```python
from build123d import *

# Parameters (mm, degrees)
BOSS_EXTRUDE1_DEPTH = 5.5
SKETCH2_R           = 1.65
CUT_EXTRUDE1_DEPTH  = 5.5
BOSS_EXTRUDE2_DEPTH = 3
CUT_EXTRUDE2_DEPTH  = 2.75
SKETCH5_R           = 1.95
SKETCH5_R_2         = 1.35
SKETCH5_R_3         = 1.15
SKETCH5_R_4         = 2
CUT_EXTRUDE3_DEPTH  = 4.3
SKETCH7_R           = 1.95
SKETCH7_R_2         = 1.35
CUT_EXTRUDE4_DEPTH  = 3
CHAMFER1_SIZE       = 1
CUT_EXTRUDE5_DEPTH  = 2.75


with BuildPart() as part:
    # Sketch1 → Boss-Extrude1 (new body)
    with BuildSketch(Plane(origin=(0, 0, 0), x_dir=(1, 0, 0), z_dir=(0, 1, 0))):
        with BuildLine():
            Line((-7.755996733, 16.049992949), (-18.008818061, 22.554712546))
            ThreePointArc((-18.008818061, 22.554712546), (-25.669699487, 29.278547542), (-27.75, 19.3))
            Line((-27.75, 19.3), (-27.75, 8.1))
            Line((-27.75, 8.1), (-21.75, 2.8))
            Line((-21.75, 2.8), (-21.75, 0))
            Line((-21.75, 0), (21.75, 0))
            Line((21.75, 0), (21.75, 7))
            Line((21.75, 7), (18.25, 11))
            Line((18.25, 11), (-5.907756778, 15.263133549))
            ThreePointArc((-5.907756778, 15.263133549), (-6.75113203, 15.846223088), (-7.755996733, 16.049992949))
        make_face()
        with BuildLine():
            Line((-19.85, 18.630440726), (-10.05956754, 12.419075498))
            ThreePointArc((-10.05956754, 12.419075498), (-8.75757921, 11.15750472), (-6.94630287, 11.079964685))
            Line((-6.94630287, 11.079964685), (-0.119008465, 9.875148026))
            Line((-0.119008465, 9.875148026), (2.380991535, 6.875148026))
            Line((2.380991535, 6.875148026), (2.380991535, 1.3))
            Line((2.380991535, 1.3), (-12.151886792, 1.3))
            Line((-12.151886792, 1.3), (-19.85, 8.1))
            Line((-19.85, 8.1), (-19.85, 18.630440726))
        make_face(mode=Mode.SUBTRACT)
    extrude(amount=BOSS_EXTRUDE1_DEPTH)

    # Sketch2 → Cut-Extrude1 (cut)
    with BuildSketch(Plane(origin=(0, 5.5, 0), x_dir=(1, 0, 0), z_dir=(0, 1, 0))):
        with Locations(Location((-7.75, 13.5, 0), (0, 0, 270))):
            Circle(SKETCH2_R)
    extrude(amount=-CUT_EXTRUDE1_DEPTH, mode=Mode.SUBTRACT)

    # Sketch3 → Boss-Extrude2 (add)
    with BuildSketch(Plane(origin=(0, 5.5, 0), x_dir=(1, 0, 0), z_dir=(0, 1, 0))):
        with BuildLine():
            ThreePointArc((-27.75, 19.3), (-23.8, 17.782636193), (-19.85, 19.3))
            ThreePointArc((-19.85, 19.3), (-18.664735174, 20.777631), (-18.008818061, 22.554712546))
            ThreePointArc((-18.008818061, 22.554712546), (-17.927267525, 23.116055854), (-17.9, 23.682636193))
            ThreePointArc((-17.9, 23.682636193), (-26.198436991, 29.073137097), (-27.75, 19.3))
        make_face()
        with BuildLine():
            Line((-12.151886792, 1.3), (-19.85, 8.1))
            Line((-19.85, 8.1), (-19.85, 18.630440726))
            Line((-19.85, 18.630440726), (-19.85, 19.3))
            ThreePointArc((-19.85, 19.3), (-23.8, 17.782636193), (-27.75, 19.3))
            Line((-27.75, 19.3), (-27.75, 8.1))
            Line((-27.75, 8.1), (-21.75, 2.8))
            Line((-21.75, 2.8), (-21.75, 0))
            Line((-21.75, 0), (21.75, 0))
            Line((21.75, 0), (21.75, 1.3))
            Line((21.75, 1.3), (2.380991535, 1.3))
            Line((2.380991535, 1.3), (-12.151886792, 1.3))
        make_face()
    extrude(amount=BOSS_EXTRUDE2_DEPTH)

    # Sketch4 → Cut-Extrude2 (cut)
    with BuildSketch(Plane.XZ):
        with BuildLine():
            ThreePointArc((-27.75, -19.3), (-29.307610804, -25.798344876), (-23.8, -29.582636193))
            Line((-23.8, -29.582636193), (-23.8, -7.3))
            Line((-23.8, -7.3), (-26.844339623, -7.3))
            Line((-26.844339623, -7.3), (-27.75, -8.1))
            Line((-27.75, -8.1), (-27.75, -19.3))
        make_face()
    extrude(amount=-CUT_EXTRUDE2_DEPTH, mode=Mode.SUBTRACT)

    # Sketch5 → Cut-Extrude3 (cut)
    with BuildSketch(Plane.XZ):
        with Locations(Location((-23.8, -23.682636193, 0), (0, 0, 90))):
            Circle(SKETCH5_R)
        with Locations(Location((-23.8, -13.882636193, 0), (0, 0, 90))):
            Circle(SKETCH5_R_2)
        with Locations(Location((-20, -4.382636193, 0), (0, 0, 270))):
            Circle(SKETCH5_R_3)
        with Locations(Location((15.000589162, -5.5, 0), (0, 0, 270))):
            Circle(SKETCH5_R_4)
    extrude(amount=-CUT_EXTRUDE3_DEPTH, mode=Mode.SUBTRACT)

    # Sketch7 → Cut-Extrude4 (cut)
    with BuildSketch(Plane.XZ.offset(-4.3)):
        with Locations(Location((-23.8, -23.682636193, 0), (0, 0, 90))):
            Circle(SKETCH7_R)
        with Locations(Location((-23.8, -13.882636193, 0), (0, 0, 90))):
            Circle(SKETCH7_R_2)
    extrude(amount=-CUT_EXTRUDE4_DEPTH, mode=Mode.SUBTRACT)

    # Chamfer1
    chamfer1_edges = [part.edges().sort_by_distance(p)[0] for p in [
        (-23.8, 8.5, -29.582636193),
        (-27.75, 8.5, -13.7),
        (-24.75, 8.5, -5.45),
        (-21.75, 8.5, -1.4),
        (-19.85, 8.5, -13.7),
    ]]
    chamfer(chamfer1_edges, length=CHAMFER1_SIZE)

    # Sketch8 → Cut-Extrude5 (cut)
    with BuildSketch(Plane.XZ):
        with BuildLine():
            Line((-21.05, -7.3), (-23.8, -7.3))
            Line((-23.8, -7.3), (-23.8, -12.532636193))
            ThreePointArc((-23.8, -12.532636193), (-22.45, -13.882636193), (-23.8, -15.232636193))
            Line((-23.8, -15.232636193), (-23.8, -18.982636193))
            ThreePointArc((-23.8, -18.982636193), (-22.355013861, -19.210274953), (-21.05, -19.871140424))
            Line((-21.05, -19.871140424), (-21.05, -7.3))
        make_face()
        with BuildLine():
            ThreePointArc((-19.1, -23.682636193), (-19.615803542, -21.54195873), (-21.05, -19.871140424))
            ThreePointArc((-21.05, -19.871140424), (-22.355013861, -19.210274953), (-23.8, -18.982636193))
            Line((-23.8, -18.982636193), (-23.8, -21.732636193))
            ThreePointArc((-23.8, -21.732636193), (-21.85, -23.682636193), (-23.8, -25.632636193))
            Line((-23.8, -25.632636193), (-23.8, -28.382636193))
            ThreePointArc((-23.8, -28.382636193), (-20.476598128, -27.006038065), (-19.1, -23.682636193))
        make_face()
        with BuildLine():
            Line((-23.8, -21.732636193), (-23.8, -18.982636193))
            ThreePointArc((-23.8, -18.982636193), (-28.5, -23.682636193), (-23.8, -28.382636193))
            Line((-23.8, -28.382636193), (-23.8, -25.632636193))
            ThreePointArc((-23.8, -25.632636193), (-21.85, -23.682636193), (-23.8, -21.732636193))
        make_face()
    extrude(amount=-CUT_EXTRUDE5_DEPTH, mode=Mode.SUBTRACT)


solid = part.part
```
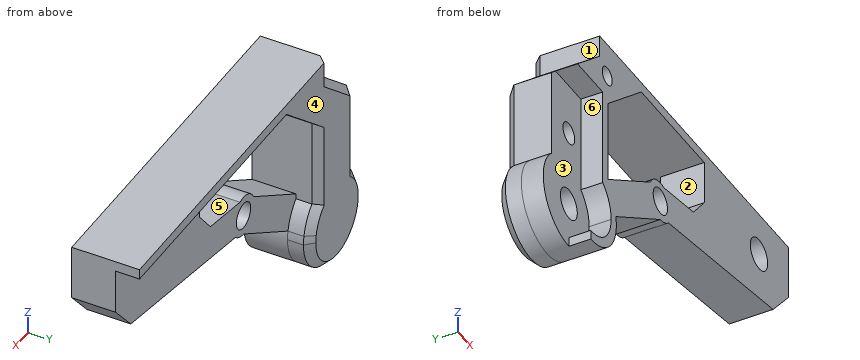
The listing builds one solid part. Answer for the finished solid, in the listing's coordinates (mm). Face numbers are marked on the shaded views. A direction names the side the tool comes from. Give positions to 0.01 mm unless a question says otherwise; leave off trailing zeros. Order: outer loops, then holes, each group sorted by start corner. A loop starts at its lowest first (then second) coordinate and runs counter-clockwise, first axis right, second up.
Item 1: The part is cut by section B-B, the plane y = 1.75. Give the vertices of the cut face in (x, z), and give its area (3 significant figures).
From the geometry:
outline: (-26.84, -7.3) - (-21.05, -7.3) - (-21.05, -19.87) arc R4.7 cw to (-23.8, -28.38) - (-23.8, -29.58) arc R5.9 ccw to (-18.01, -22.55) - (-7.76, -16.05) arc R2.55 ccw to (-5.91, -15.26) - (18.25, -11) - (21.75, -7) - (21.75, 0) - (-21.75, 0) - (-21.75, -2.8) - close; hole circle Ø2.3 at (-20, -4.38); hole (-19.85, -18.63) - (-10.06, -12.42) arc R2.55 cw to (-6.95, -11.08) - (-0.12, -9.88) - (2.38, -6.88) - (2.38, -1.3) - (-12.15, -1.3) - (-19.85, -8.1) - close; hole circle Ø3.3 at (-7.75, -13.5); hole circle Ø4 at (15, -5.5)
area: 420 mm2
Item 2: The part is cut by section A-A, the plane z = -13.5. Give the vertices of the cut face in (x, y), and give its area (3 significant figures).
From the geometry:
outline: (-27.75, 2.75) - (-25.09, 2.75) - (-25.09, 7.3) - (-22.51, 7.3) - (-22.51, 2.75) - (-21.05, 2.75) - (-21.05, 0) - (-19.85, 0) - (-19.85, 7.5) - (-20.85, 8.5) - (-26.75, 8.5) - (-27.75, 7.5) - close; (-11.76, 0) - (-9.4, 0) - (-9.4, 5.5) - (-11.76, 5.5) - close; (-6.1, 0) - (4.08, 0) - (4.08, 5.5) - (-6.1, 5.5) - close
area: 105 mm2
Item 3: The part is cut by section C-C, the plane x = 5.5. Give the vertices of the cut face in (y, z).
From the geometry:
outline: (0, -13.25) - (5.5, -13.25) - (5.5, -1.3) - (8.5, -1.3) - (8.5, 0) - (0, 0) - close
Item 4: Find the intervals of material crossed by probe 1 along Z at (x, y) = (-23.8, 4.35); probe 2 along X at (y, z) = (6.5, -23.5); probe 3 along Y at (x, z) = (-10.5, -12.75), in increasing order.
From the geometry:
probe 1: z = -29.58 to -25.63, -21.73 to -15.23, -12.53 to -4.61
probe 2: x = -29.7 to -25.74, -21.86 to -17.9
probe 3: y = 0 to 5.5
Item 5: Given pin 1 Ø1.4 at (y, z) = (1, -12.5) entering from -X; pin 2 Ø3 at (x, z) = (15, -4.5) entering from -Y; pin 3 Ø5.5 at (x, z) = (-23, -24) entering from -Y; pin 4 Ø6 at (x, z) = (1.5, -20) entering from -Y, each flat-ended and moving along its own axis, determine where each tip first touches the part or whether it passes through.
From the geometry:
pin 1: stops at x = -21.05
pin 2: stops at y = 0
pin 3: stops at y = 2.75
pin 4: passes through
Item 6: Which of the six approach directions +Z, -Z, +X, -X, +Y, -Y give full straight-line access (tool end or side, diameter ignored) to the marked faces 1, 2 and 3?
From the geometry:
face 1: +Z, -X, +Y, -Y
face 2: +Y, -Y
face 3: -X, -Y
Item 7: For a pull along X with two mould halves and no side action, classify the marked faces 4, 5 and 6 as pulls with the +X half, pulls with the -X half, needs draft (parallel to the pull), parting line crosses it, or undercut.
From the geometry:
face 4: needs draft
face 5: undercut
face 6: pulls with the -X half
